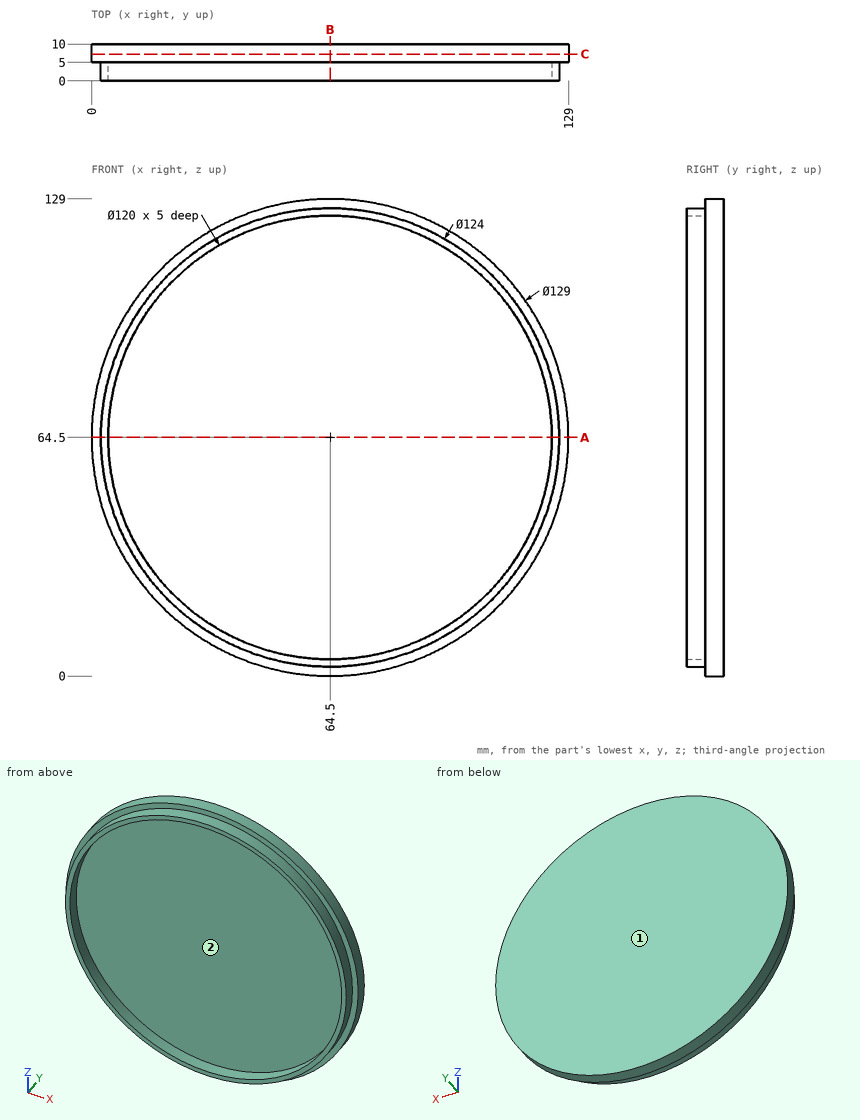
Job drawing, mm, ordinate dimensions from the low corner. One solid piece. Round coordinates to 2 decimals unless told otherwise and drop trailing zeros. Write each loop counter-clockwise with the first axis right and the second up, starting at its lowest first coordinate (ties: lowest second). Pieces come first, ordered by that corner, then holes. Notation, with made-up numbers: M 14,39.25 L 18,39.25 A25 cw 18,56.25 Z; hole C 36,11.25 d10. An arc over 180 degrees is marked long. Return JSON: item names as keys, results as strings. Group by question number.
(1) Drill centre lines: probe 1 along X at (y, z) = (1.35, 64.5); probe 2 along Y at (x, z) = (48, 53.5). Where is each one in solid material? Low to high.
(2) Saw through at A-A on z = 64.5. Write the cut outline in (x, y).
(3) Pin check, flat tips, straight feed: pin 1 Ø2 at (x, z) = (54.5, 100.5) entering from -Y; pin 2 Ø6 at (x, y) = (103, 6) entering from -Z; pin 3 Ø1 at (x, y) = (30, 5.5) entering from -Z. Stop position of each tip, or through.
(4) Saw through at B-B on x = 64.5. Write the cut outline in (y, z).
(5) Saw through at C-C on y = 7.25. Write the cut outline in (x, z), then the cut area to 3 significant figures.
(6) Two-plate mould, pull along Z, no slides. Class the marked faces 1 and 2: +Z half, -Z half, draft (parallel to the pull), parting line (faces both ways), or undercut.
Returned:
{
 "1": {"probe 1": "2.5 to 4.5, 124.5 to 126.5", "probe 2": "5 to 10"},
 "2": {"outline": "M 0,5 L 2.5,5 L 2.5,0 L 4.5,0 L 4.5,5 L 124.5,5 L 124.5,0 L 126.5,0 L 126.5,5 L 129,5 L 129,10 L 0,10 Z"},
 "3": {"pin 1": "y = 5", "pin 2": "z = 10.65", "pin 3": "z = 9.69"},
 "4": {"outline": "M 0,2.5 L 5,2.5 L 5,0 L 10,0 L 10,129 L 5,129 L 5,126.5 L 0,126.5 L 0,124.5 L 5,124.5 L 5,4.5 L 0,4.5 Z"},
 "5": {"outline": "C 64.5,64.5 d129", "area": "13,100 mm²"},
 "6": {"face 1": "draft", "face 2": "undercut"}
}
